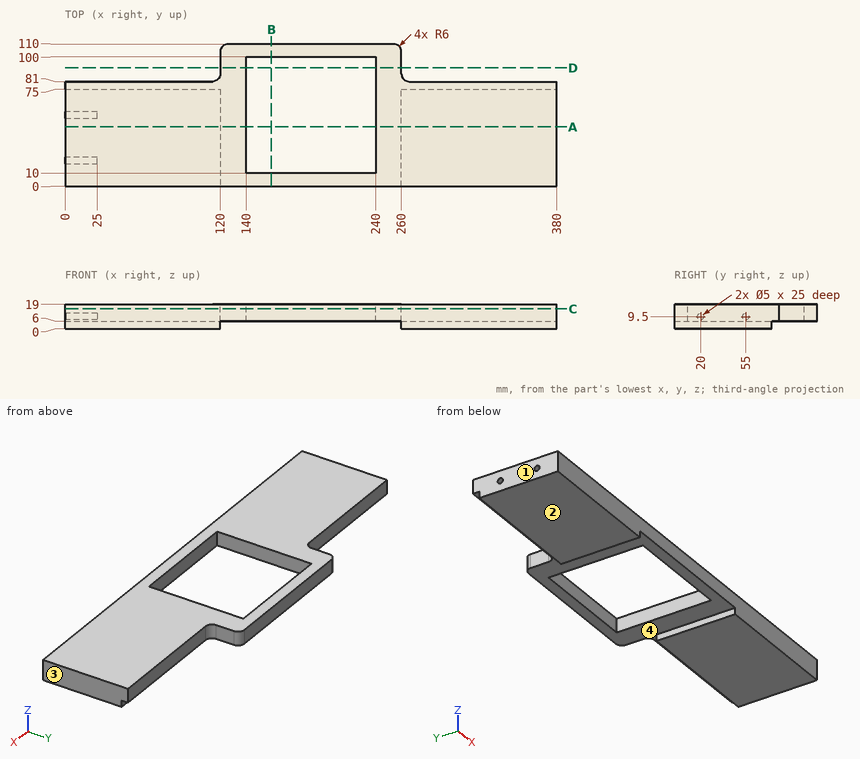
Source: three-view drawing plus pictorial views. Frame: mm from the lowest corner of the part. Round coordinates to 2 decimals unless told otherwise and drop trailing zeros. Order: outer loops, then holes, each group sorted by start corner. A loop starts at its lowest first (then second) coordinate and runs counter-clockwise, first axis right, second up. Notation, with made-up numbers: (2.25, 49.5) -> (31.25, 49.5) arc R14 cw to (31.25, 53.5) -> close; hole circle Ø5 at (76, 65.5). An arc over 180 degrees is marked (long way). Use one line per item in the form item = value. Start each with the question number.
1. Cut plane D-D (y = 91.5). Return the cut outline in (x, z).
2. Cut plane A-A (y = 46). Return the cut outline in (x, z).
3. Draft query along X for the marked faces 1, 2, 3 and 4. Return one class per face: pulls with the +X half, pulls with the -X half, needs draft (parallel to the pull), parting line crosses it, or undercut.
4. Cut plane B-B (x = 159.5). Return the cut outline in (y, z), then the cut area to 3 significant figures.
5. Line query: probe 1 along Z at (x, y) = (15, 20); probe 2 along X at (y, z) = (58, 1); probe 3 along X at (y, z) = (46.5, 14). Output: solid intervals per line, ascending.
6. Pin query (flat end, axial travel): pin 1 Ø4 at (x, z) = (299.5, 10) entering from +Y; pin 2 Ø6.5 at (x, z) = (65.5, 2.5) entering from +Y; pin 3 Ø1.5 at (y, z) = (19, 14.5) entering from -X; pin 4 Ø10.5 at (y, z) = (97, 15) entering from -X. Return the tip coordinate at first contact, or that it passes through.
7. Cut plane C-C (z = 15.5). Return the cut outline in (x, y).
Solution:
q1.outline = (120, 6) -> (140, 6) -> (140, 19) -> (120, 19) -> close; (240, 6) -> (260, 6) -> (260, 19) -> (240, 19) -> close
q2.outline = (0, 0) -> (120, 0) -> (120, 6) -> (140, 6) -> (140, 19) -> (0, 19) -> close; (240, 6) -> (260, 6) -> (260, 0) -> (380, 0) -> (380, 19) -> (240, 19) -> close
q3.face_1 = pulls with the -X half
q3.face_2 = needs draft
q3.face_3 = pulls with the +X half
q3.face_4 = undercut
q4.outline = (0, 6) -> (10, 6) -> (10, 19) -> (0, 19) -> close; (100, 6) -> (110, 6) -> (110, 19) -> (100, 19) -> close
q4.area = 260 mm^2
q5.probe_1 = 0 to 7, 12 to 19
q5.probe_2 = 0 to 120, 260 to 380
q5.probe_3 = 0 to 140, 240 to 380
q6.pin_1 = 81
q6.pin_2 = 75
q6.pin_3 = 0
q6.pin_4 = 120
q7.outline = (0, 0) -> (380, 0) -> (380, 81) -> (266, 81) arc R6 cw to (260, 87) -> (260, 104) arc R6 ccw to (254, 110) -> (126, 110) arc R6 ccw to (120, 104) -> (120, 87) arc R6 cw to (114, 81) -> (0, 81) -> close; hole (140, 10) -> (240, 10) -> (240, 100) -> (140, 100) -> close
